Can you work these out from the model? Positions are in its coordinate system, mm. A direction names the side the tool comes from. Coordinates: 2 decimals unless noted, no trailing zeros. Write each loop counter-clockwise with the first axis right and the second up, starting at its lowest first coordinate (ties: lowest second). Pieces come first, ordered by that corner, then holes.
```python
from build123d import *

# Parameters (mm, degrees)
SKETCH_1_W          = 109.5
SKETCH_1_H          = 60
EXTRUDE_1_DEPTH     = 3
SKETCH_2_R          = 1.25
CUT_EXTRUDE_1_DEPTH = 10
FILLET_1_R          = 3
CUT_EXTRUDE_2_DEPTH = 10
SKETCH_5_R          = 7.5
CUT_EXTRUDE_3_DEPTH = 10


with BuildPart() as part:
    # 草图1 → 凸台-拉伸1 (new body)
    with BuildSketch(Plane(origin=(0, 0, 0), x_dir=(1, 0, 0), z_dir=(0, 1, 0))):
        Rectangle(SKETCH_1_W, SKETCH_1_H)
    extrude(amount=EXTRUDE_1_DEPTH)

    # 草图2 → 切除-拉伸1 (cut)
    with BuildSketch(Plane(origin=(0, 3, 0), x_dir=(1, 0, 0), z_dir=(0, 1, 0))):
        with Locations((9, -26)):
            Circle(SKETCH_2_R)
        with Locations((-9, -26)):
            Circle(SKETCH_2_R)
    extrude(amount=-CUT_EXTRUDE_1_DEPTH, mode=Mode.SUBTRACT)

    # 圆角1
    fillet_1_edges = [part.edges().sort_by_distance(p)[0] for p in [
        (54.75, 1.5, 30),
        (-54.75, 1.5, 30),
        (-54.75, 1.5, -30),
        (54.75, 1.5, -30),
    ]]
    fillet(fillet_1_edges, radius=FILLET_1_R)

    # 草图3 → 切除-拉伸2 (cut)
    with BuildSketch(Plane(origin=(0, 3, 0), x_dir=(1, 0, 0), z_dir=(0, 1, 0))):
        with BuildLine():
            Line((-43.809910809, 5), (-43.809910809, -5))
            ThreePointArc((-43.809910809, -5), (-46, -7.190089191), (-48.190089191, -5))
            Line((-48.190089191, -5), (-48.190089191, 5))
            ThreePointArc((-48.190089191, 5), (-46, 7.190089191), (-43.809910809, 5))
        make_face()
        with BuildLine():
            Line((43.809910809, 5), (43.809910809, -5))
            ThreePointArc((43.809910809, -5), (46, -7.190089191), (48.190089191, -5))
            Line((48.190089191, -5), (48.190089191, 5))
            ThreePointArc((48.190089191, 5), (46, 7.190089191), (43.809910809, 5))
        make_face()
    extrude(amount=-CUT_EXTRUDE_2_DEPTH, mode=Mode.SUBTRACT)

    # 草图5 → 切除-拉伸3 (cut)
    with BuildSketch(Plane(origin=(0, 3, 0), x_dir=(1, 0, 0), z_dir=(0, 1, 0))):
        with Locations((22, 10)):
            Circle(SKETCH_5_R)
        with BuildLine():
            Line((-26.5, 15), (-26.5, -15))
            ThreePointArc((-26.5, -15), (-28, -16.5), (-29.5, -15))
            Line((-29.5, -15), (-29.5, 15))
            ThreePointArc((-29.5, 15), (-28, 16.5), (-26.5, 15))
        make_face()
        with BuildLine():
            Line((-16.5, 15), (-16.5, -15))
            ThreePointArc((-16.5, -15), (-18, -16.5), (-19.5, -15))
            Line((-19.5, -15), (-19.5, 15))
            ThreePointArc((-19.5, 15), (-18, 16.5), (-16.5, 15))
        make_face()
        with BuildLine():
            Line((-6.5, 15), (-6.5, -15))
            ThreePointArc((-6.5, -15), (-8, -16.5), (-9.5, -15))
            Line((-9.5, -15), (-9.5, 15))
            ThreePointArc((-9.5, 15), (-8, 16.5), (-6.5, 15))
        make_face()
        with BuildLine():
            Line((3.5, 15), (3.5, -15))
            ThreePointArc((3.5, -15), (2, -16.5), (0.5, -15))
            Line((0.5, -15), (0.5, 15))
            ThreePointArc((0.5, 15), (2, 16.5), (3.5, 15))
        make_face()
    extrude(amount=-CUT_EXTRUDE_3_DEPTH, mode=Mode.SUBTRACT)


solid = part.part
```
1. If I drill on L1, parallel to X at y = 1.45, z = 11.5; L2, parallel to X at y = 1.9, z = -10; L3, parallel to X at y = 1.25, z = 26, over which ranges is the centre line in solid material (lowest first)?
2. If we section it at B-B, the plane y = 0.5: Count the separate pieces of the cut face and the enclosed holes in it, plus the area to 3 significant figures.
3. Which directions (+Z, -Z, +X, -X, +Y, -Y) give clear straight access to the entire face, cutting with the end or side of a thin tool? Please do faces 1 (the face through (45.95, 1.52, 7.19)), 2 (the face through (-1, 1, -30)).
4. If we section it at C-C, the plane x = -28: List the corners of the cut face in (y, z) for me, plus the area to 3 significant figures.
5. We'd pull the mould along X, two halves only. Please class faces 3 (the face through (-1, 3, 0)), 4 (the face through (48.19, 2, 0)), 5 (the face through (53.85, 1.52, -29.14)), 6 (the face through (-9.99, 1.52, 26.76)): released by +X, released by -X, zero draft, split by the parting line, or undercut.
6. If we section it at A-A, the plane x = -46: List the corners of the cut face in (y, z) for me.
7. I'm going to push a flat-ended pin straight in: P1, Ø9, axis at x = 22, z = -10, coming from the +Y side. Where does the tip first touch, or does it pass through?
Answers:
1. L1: x = -54.75 to -29.5, -26.5 to -19.5, -16.5 to -9.5, -6.5 to 0.5, 3.5 to 54.75
1. L2: x = -54.75 to -29.5, -26.5 to -19.5, -16.5 to -9.5, -6.5 to 0.5, 3.5 to 14.5, 29.5 to 54.75
1. L3: x = -54.75 to -10.25, -7.75 to 7.75, 10.25 to 54.75
2. separate pieces: 1
2. enclosed holes: 9
2. area: 5,870 mm2
3. face 1: +Y, -Y
3. face 2: -Z, +X, -X, +Y, -Y
4. outline: (0, -30) - (3, -30) - (3, -16.5) - (0, -16.5) - close; (0, 16.5) - (3, 16.5) - (3, 30) - (0, 30) - close
4. area: 81.0 mm2
5. face 3: zero draft
5. face 4: undercut
5. face 5: released by +X
5. face 6: undercut
6. outline: (0, -30) - (3, -30) - (3, -7.19) - (0, -7.19) - close; (0, 7.19) - (3, 7.19) - (3, 30) - (0, 30) - close
7. P1: passes through
